```python
from build123d import *

# Parameters (mm, degrees)
BOX_W             = 10
BOX_H             = 10
BOX_DEPTH         = 10
SKETCH_W          = 4.4
SKETCH_H          = 4.4
PAD_DEPTH         = 4
PAD_FACE1_W       = 10
PAD_FACE1_H       = 10
POCKET_DEPTH      = 2.5
POCKET_FACE3_W    = 10
POCKET_FACE3_H    = 10
POCKET001_DEPTH   = 2.5
POCKET001_FACE6_W = 5
POCKET001_FACE6_H = 10
PAD001_DEPTH      = 10
SKETCH001_W       = 4.4
SKETCH001_H       = 4.4
PAD002_DEPTH      = 4
PAD002_FACE14_W   = 5
PAD002_FACE14_H   = 10
PAD003_DEPTH      = 10
SKETCH002_W       = 4.4
SKETCH002_H       = 4.4
PAD004_DEPTH      = 4


with BuildPart() as part:
    # Box → Box (new body)
    with BuildSketch(Plane.XY):
        with Locations((5, 5)):
            Rectangle(BOX_W, BOX_H)
    extrude(amount=BOX_DEPTH)

    # Sketch (on Face6 of BaseFeature) → Pad (new body)
    with BuildSketch(Plane.XY.offset(10)):
        with Locations((5, 5)):
            Rectangle(SKETCH_W, SKETCH_H)
    extrude(amount=PAD_DEPTH)

    # Pad Face1 → Pocket (cut)
    with BuildSketch(Plane(origin=(0, 5, 5), x_dir=(0, 1, 0), z_dir=(-1, 0, 0))):
        Rectangle(PAD_FACE1_W, PAD_FACE1_H)
    extrude(amount=-POCKET_DEPTH, mode=Mode.SUBTRACT)

    # Pocket Face3 → Pocket001 (cut)
    with BuildSketch(Plane(origin=(10, 5, 5), x_dir=(0, -1, 0), z_dir=(1, 0, 0))):
        Rectangle(POCKET_FACE3_W, POCKET_FACE3_H)
    extrude(amount=-POCKET001_DEPTH, mode=Mode.SUBTRACT)

    # Pocket001 Face6 → Pad001 (add)
    with BuildSketch(Plane(origin=(5, 10, 5), x_dir=(1, 0, 0), z_dir=(0, 1, 0))):
        Rectangle(POCKET001_FACE6_W, POCKET001_FACE6_H)
    extrude(amount=PAD001_DEPTH)

    # Sketch001 (on Face8 of Pad001) → Pad002 (join)
    with BuildSketch(Plane.XY.offset(10)):
        with Locations((5, 15)):
            Rectangle(SKETCH001_W, SKETCH001_H)
    extrude(amount=PAD002_DEPTH)

    # Pad002 Face14 → Pad003 (add)
    with BuildSketch(Plane(origin=(5, 20, 5), x_dir=(1, 0, 0), z_dir=(0, 1, 0))):
        Rectangle(PAD002_FACE14_W, PAD002_FACE14_H)
    extrude(amount=PAD003_DEPTH)

    # Sketch002 (on Face16 of Pad003) → Pad004 (join)
    with BuildSketch(Plane.XY.offset(10)):
        with Locations((5, 25)):
            Rectangle(SKETCH002_W, SKETCH002_H)
    extrude(amount=PAD004_DEPTH)


solid = part.part
```
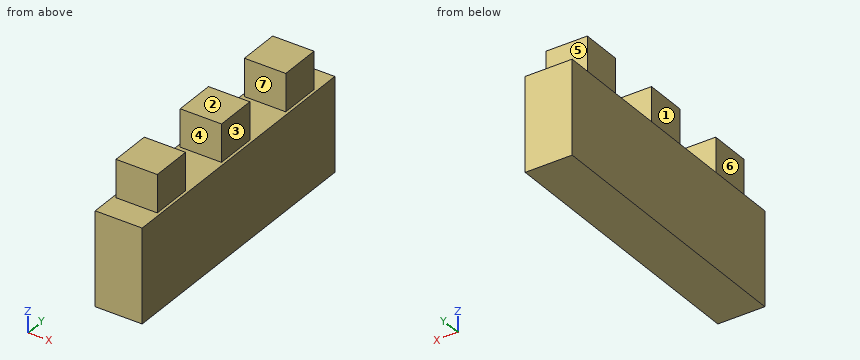
CAD build for the part. Positions are in the model's coordinates, mm. Face numbers are marked on the shaded views. A direction names the side the tool comes from. Coordinates: 2 decimals unless noted, no trailing zeros. Order: outer loops, then holes, each group sorted by start corner. A loop starts at its lowest first (then second) coordinate and runs counter-clockwise, first axis right, second up. Notation, with made-up numbers: (-31, 67.5) - (-26, 67.5) arc R31 ccw to (-26, 96.5) - close; hole circle Ø7 at (85, 52.5). An arc over 180 degrees is marked (long way). Use a Markdown table: item, result. Add a question column.
(1) Drill centre lines: line 1 along Y through (x, z) = (5.2, 10.5); line 2 along Z through (x, y) = (4.15, 7.5); line 3 along X through (y, z) = (24, 11). Where is each one in solid material? Low to high. Write a range as [from, to].
(2) Saw through at A-A (z = 13). Give the cut face in (x, y).
(3) Saw through at D-D (y = 12.25). Give the cut face in (x, z), then the cut area to 3 significant figures.
(4) Saw through at B-B (x = 6.1). Give the cut face in (y, z), then the cut area to 3 significant figures.
(5) Which spindle directions (+Z, -Z, +X, -X, +Y, -Y) get a long thin tool onto all of the face, cutting with end or side? Do the marked faces 1, 2 and 3. Say none if no direction does.
(6) Flat gauge pins, fed straight in: pin 1 (2 mm diameter, centred on y = 14, z = 13, fed in from +X); pin 2 (1.2 mm diameter, centred on x = 5.5, z = 12.5, fed in from +Y); pin 3 (3 mm diameter, centred on y = 25, z = 12, fed in from -X). Where does each tip first touch, or does it go through?
(7) Pull direction Y, two halves, no side cores. Call the marked faces 4, 5, 6 and 7: +Y half, -Y half, draft (parallel to the pull), parting line (faces both ways), or undercut.
(8) Saw through at C-C (y = 5.5). Give the cut face in (x, z).
Solved:
| question | item | result |
|---|---|---|
| 1 | line 1 | y = [2.8, 7.2], [12.8, 17.2], [22.8, 27.2] |
| 1 | line 2 | z = [0, 10] |
| 1 | line 3 | x = [2.8, 7.2] |
| 2 | outline | (2.8, 2.8) - (7.2, 2.8) - (7.2, 7.2) - (2.8, 7.2) - close; (2.8, 12.8) - (7.2, 12.8) - (7.2, 17.2) - (2.8, 17.2) - close; (2.8, 22.8) - (7.2, 22.8) - (7.2, 27.2) - (2.8, 27.2) - close |
| 3 | outline | (2.5, 0) - (7.5, 0) - (7.5, 10) - (2.5, 10) - close |
| 3 | area | 50.0 mm² |
| 4 | outline | (0, 0) - (30, 0) - (30, 10) - (27.2, 10) - (27.2, 14) - (22.8, 14) - (22.8, 10) - (17.2, 10) - (17.2, 14) - (12.8, 14) - (12.8, 10) - (7.2, 10) - (7.2, 14) - (2.8, 14) - (2.8, 10) - (0, 10) - close |
| 4 | area | 353 mm² |
| 5 | face 1 | +Z, -X, +Y, -Y |
| 5 | face 2 | +Z, +X, -X, +Y, -Y |
| 5 | face 3 | +Z, +X, +Y, -Y |
| 6 | pin 1 | stops at x = 7.2 |
| 6 | pin 2 | stops at y = 27.2 |
| 6 | pin 3 | stops at x = 2.8 |
| 7 | face 4 | undercut |
| 7 | face 5 | +Y half |
| 7 | face 6 | draft |
| 7 | face 7 | undercut |
| 8 | outline | (2.5, 0) - (7.5, 0) - (7.5, 10) - (7.2, 10) - (7.2, 14) - (2.8, 14) - (2.8, 10) - (2.5, 10) - close |
